Model file for the job. Use its own axes, mm. Face numbers are marked on the shaded views. A direction names the side the tool comes from. Round coordinates to 2 decimals unless told otherwise and drop trailing zeros. Order: outer loops, then holes, each group sorted by start corner. A loop starts at its lowest first (then second) coordinate and runs counter-clockwise, first axis right, second up. Notation, with made-up numbers: (-23, 0) -> (16, 0) arc R16 cw to (16, 17) -> close; hole circle Ø4 at (80.5, -20.5). An arc over 180 degrees is marked (long way). Use CSV: the item, a comma, the result in double quotes.
```python
from build123d import *

# Parameters (mm, degrees)
SKETCH2_R           = 22.5
BOSS_EXTRUDE1_DEPTH = 5
SKETCH3_R           = 2
CUT_EXTRUDE1_DEPTH  = 5
SKETCH4_R           = 4
CUT_EXTRUDE2_DEPTH  = 10


with BuildPart() as part:
    # Sketch2 → Boss-Extrude1 (new body)
    with BuildSketch(Plane.XY):
        Circle(SKETCH2_R)
        Polygon((-22.5, 0), (-2.5, -22.360679775), (-24.860679775, -42.360679775), (-44.860679775, -20), align=None)
        Polygon((2.5, -22.360679775), (22.5, 0), (44.860679775, -20), (24.860679775, -42.360679775), align=None)
    extrude(amount=BOSS_EXTRUDE1_DEPTH)

    # Sketch3 → Cut-Extrude1 (cut)
    with BuildSketch(Plane(origin=(0, 0, 0), x_dir=(-1, 0, 0), z_dir=(0, 0, -1))):
        with Locations((-37.800566479, -20.393446629)):
            Circle(SKETCH3_R)
        with Locations((-22.893446629, -7.060113296)):
            Circle(SKETCH3_R)
        with Locations((-9.560113296, -21.967233146)):
            Circle(SKETCH3_R)
        with Locations((-24.467233146, -35.300566479)):
            Circle(SKETCH3_R)
        with Locations((24.467233146, -35.300566479)):
            Circle(SKETCH3_R)
        with Locations((37.800566479, -20.393446629)):
            Circle(SKETCH3_R)
        with Locations((9.560113296, -21.967233146)):
            Circle(SKETCH3_R)
        with Locations((22.893446629, -7.060113296)):
            Circle(SKETCH3_R)
    extrude(amount=-CUT_EXTRUDE1_DEPTH, mode=Mode.SUBTRACT)

    # Sketch4 → Cut-Extrude2 (cut)
    with BuildSketch(Plane(origin=(0, 0, 0), x_dir=(-1, 0, 0), z_dir=(0, 0, -1))):
        with Locations((0, 10)):
            Circle(SKETCH4_R)
    extrude(amount=-CUT_EXTRUDE2_DEPTH, mode=Mode.SUBTRACT)


solid = part.part
```
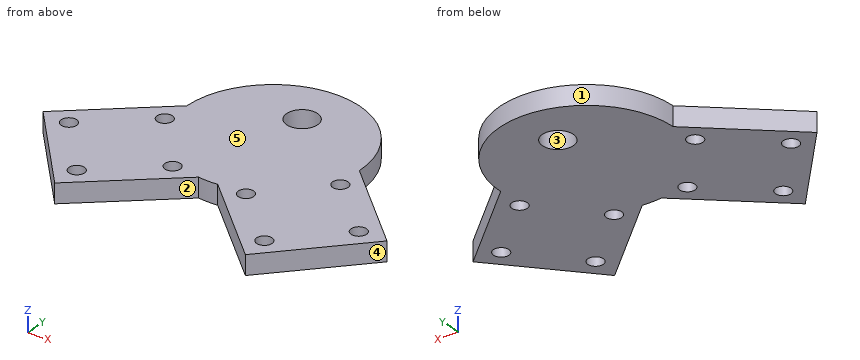
Q1. Cut at B-B (y = 10). Give the cut face in (x, z).
From the geometry:
outline,"(-20.16, 0) -> (-4, 0) -> (-4, 5) -> (-20.16, 5) -> close; (4, 0) -> (20.16, 0) -> (20.16, 5) -> (4, 5) -> close"
Q2. Pin check, flat tips, straight feed: pin 1 (2 mm diameter, centred on y = -1.5, z = 1, fed in from -X); pin 2 (4.5 mm diameter, centred on x = -22.89, y = -7.06, fed in from +Z); pin 3 (2 mm diameter, centred on x = 31, z = 3, fed in from +Y); pin 4 (3 mm diameter, centred on x = -24.47, y = -35.3, fed in from -Z). Stop position of each tip, or through.
From the geometry:
pin 1,"stops at x = -25.3"
pin 2,"stops at z = 5"
pin 3,"stops at y = -6.71"
pin 4,"passes through"
Q3. Which spindle directions (+Z, -Z, +X, -X, +Y, -Y) get a long thin tool onto all of the face, cutting with end or side? Do the marked faces 1 and 2. Say none if no direction does.
From the geometry:
face 1,"+Z, -Z, +Y"
face 2,"+Z, -Z, -Y"
Q4. Mould opens along Y. For the marked faces 3, 4 and 5 say: +Y half, -Y half, draft (parallel to the pull), parting line (faces both ways), or undercut.
From the geometry:
face 3,"undercut"
face 4,"-Y half"
face 5,"draft"
Q5. Probe line 1 along X through (y, z) = (-35, 3.65); line 2 along X through (y, z) = (-7.5, 0.95); line 3 along X through (y, z) = (-34, 3.6). List the from-to ranges inside material, lowest first.
From the geometry:
line 1,"x = -31.44 to -26.44, -22.49 to -16.63, 16.63 to 22.49, 26.44 to 31.44"
line 2,"x = -30.89 to -24.84, -20.94 to 20.94, 24.84 to 30.89"
line 3,"x = -32.34 to -25.99, -22.95 to -15.51, 15.51 to 22.95, 25.99 to 32.34"
Q6. Cut at D-D (z = 3.5). State how many separate pieces and enclosed holes the cut face has, plus the area to 3 significant figures.
From the geometry:
separate pieces,"1"
enclosed holes,"9"
area,"3,000 mm²"
Q7. Cut at C-C (y = -6). Give the cut face in (x, z), plus the area to 3 significant figures.
From the geometry:
outline,"(-29.21, 0) -> (-24.59, 0) -> (-24.59, 5) -> (-29.21, 5) -> close; (-21.2, 0) -> (21.2, 0) -> (21.2, 5) -> (-21.2, 5) -> close; (24.59, 0) -> (29.21, 0) -> (29.21, 5) -> (24.59, 5) -> close"
area,"258 mm²"
Q8. Cut at A-A (x = 0). Give the cut face in (y, z).
From the geometry:
outline,"(-22.5, 0) -> (6, 0) -> (6, 5) -> (-22.5, 5) -> close; (14, 0) -> (22.5, 0) -> (22.5, 5) -> (14, 5) -> close"
